Part model, mm, in its own coordinate system. Face numbers are marked on the shaded views. A direction names the side the tool comes from. Give positions to 0.01 mm unless a question says otherwise; leave off trailing zeros. Order: outer loops, then holes, each group sorted by start corner. A loop starts at its lowest first (then second) coordinate and runs counter-clockwise, first axis right, second up. Notation, with made-up numbers: (53.5, 16.5) - (67.5, 16.5) arc R23 cw to (67.5, 50.5) - close; hole circle Ø9 at (61, -40). An arc over 180 degrees is marked (long way). Use one line per item in the form item = value. Start each with the question number.
1. Drill centre lines: line 1 (Y direction, x = -30, z = 7.2) (3 decimals); line 2 (Y direction, x = 30, z = 3.05); line 3 (X direction, y = -5, z = 5.75). Where is each one in solid material? Low to high.
2. Pull direction X, two halves, no side cores. Call the marked faces 3, 4, 5 and 6: +X half, -X half, draft (parallel to the pull), parting line (faces both ways), or undercut.
3. Pin check, flat tip, straight feed: P1, Ø7.5, axis at x = -30, y = 0, coming from the +Z side. Stop position of the tip, or through.
4. Tool access for the marked faces 1 and 2: list every direction of +Z, -Z, +X, -X, +Y, -Y with a clear straight run to the whole face (end or side of a thin tool).
5. Band-saw the part on A-A, the plane x = -30. List the corners of the cut face in (y, z) (3 decimals), plus the area to 3 significant figures.
6. Band-saw the part on C-C, the plane z = 3. List the corners of the cut face in (x, y).
7. Band-saw the part on D-D, the plane y = -8.5. List the corners of the cut face in (x, z).
8. Band-saw the part on B-B, the plane y = 0. List the corners of the cut face in (x, z) (3 decimals), plus the area to 3 significant figures.
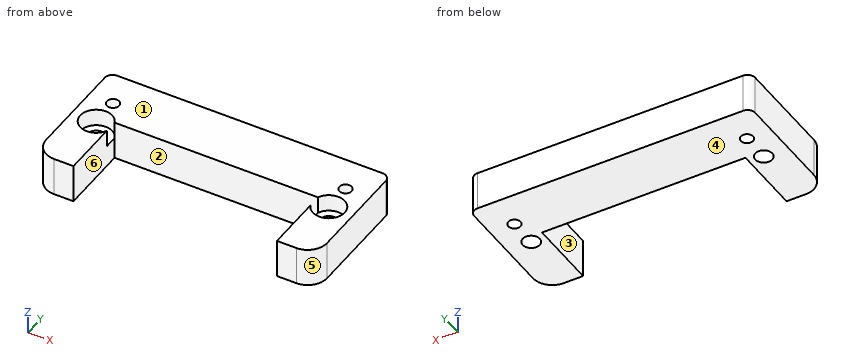
from build123d import *

# Parameters (mm, degrees)
F1_DEPTH       = 10
F3_D           = 3.2
F3_DEPTH       = 14.25
F3_TIP         = 0.9613769904
F4_R           = 5
F5_R           = 2
F7_D           = 4.4
F7_CBORE_D     = 8.25
F7_CBORE_DEPTH = 4.4


with BuildPart() as f1:
    # F0 (on Top) → F1 (new body)
    with BuildSketch(Plane.XY):
        Polygon((-36.25, 16.35), (-36.25, -16.35), (-26.25, -16.35), (-26.25, 1.65), (26.25, 1.65), (26.25, -16.35), (36.25, -16.35), (36.25, 16.35), align=None)
    extrude(amount=F1_DEPTH)

    # F3
    with Locations(Plane.XY.offset(10)):
        with Locations((-30, 7.35), (30, 7.35)):
            Hole(F3_D / 2, depth=F3_DEPTH)
            with Locations((0, 0, -(F3_DEPTH + F3_TIP / 2))):  # 118° drill point
                Cone(0, F3_D / 2, F3_TIP, mode=Mode.SUBTRACT)

    # F4
    f4_edges = [f1.edges().sort_by_distance(p)[0] for p in [
        (-36.25, -16.35, 5),
        (36.25, -16.35, 5),
    ]]
    fillet(f4_edges, radius=F4_R)

    # F5
    f5_edges = [f1.edges().sort_by_distance(p)[0] for p in [
        (36.25, 16.35, 5),
        (-36.25, 16.35, 5),
    ]]
    fillet(f5_edges, radius=F5_R)

    # F7 (through all)
    with Locations(Plane.XY.offset(10)):
        with Locations((-30, 0), (30, 0)):
            CounterBoreHole(F7_D / 2, F7_CBORE_D / 2, F7_CBORE_DEPTH)


solid = f1.part
From the geometry:
q1.line_1 = -16.35 to -4.125, 4.125 to 5.75, 8.95 to 16.35
q1.line_2 = -16.35 to -2.2, 2.2 to 5.75, 8.95 to 16.35
q1.line_3 = -36.25 to -26.25, 26.25 to 36.25
q2.face_3 = undercut
q2.face_4 = draft
q2.face_5 = +X half
q2.face_6 = undercut
q3.P1 = 5.6
q4.face_1 = +Z, +X, -X, +Y, -Y
q4.face_2 = +Z, -Z, -Y
q5.outline = (-16.35, 0) - (-2.2, 0) - (-2.2, 5.6) - (-4.125, 5.6) - (-4.125, 10) - (-16.35, 10) - close; (2.2, 0) - (5.75, 0) - (5.75, 10) - (4.125, 10) - (4.125, 5.6) - (2.2, 5.6) - close; (8.95, 0) - (16.35, 0) - (16.35, 10) - (8.95, 10) - close
q5.area = 234 mm²
q6.outline = (-36.25, -11.35) arc R5 ccw to (-31.25, -16.35) - (-26.25, -16.35) - (-26.25, 1.65) - (26.25, 1.65) - (26.25, -16.35) - (31.25, -16.35) arc R5 ccw to (36.25, -11.35) - (36.25, 14.35) arc R2 ccw to (34.25, 16.35) - (-34.25, 16.35) arc R2 ccw to (-36.25, 14.35) - close; hole circle Ø4.4 at (-30, 0); hole circle Ø3.2 at (-30, 7.35); hole circle Ø4.4 at (30, 0); hole circle Ø3.2 at (30, 7.35)
q7.outline = (-36.25, 0) - (-26.25, 0) - (-26.25, 10) - (-36.25, 10) - close; (26.25, 0) - (36.25, 0) - (36.25, 10) - (26.25, 10) - close
q8.outline = (-36.25, 0) - (-32.2, 0) - (-32.2, 5.6) - (-34.125, 5.6) - (-34.125, 10) - (-36.25, 10) - close; (-27.8, 0) - (-26.25, 0) - (-26.25, 5.6) - (-27.8, 5.6) - close; (26.25, 0) - (27.8, 0) - (27.8, 5.6) - (26.25, 5.6) - close; (32.2, 0) - (36.25, 0) - (36.25, 10) - (34.125, 10) - (34.125, 5.6) - (32.2, 5.6) - close
q8.area = 81.4 mm²
